Autodesk Inventor part; units mm, degrees
ref_plane "YZ Plane" through (0, 0, 0) normal (1, 0, 0) x (0, 1, 0)
ref_plane "XZ Plane" through (0, 0, 0) normal (0, 1, 0) x (-1, 0, 0)
ref_plane "XY Plane" through (0, 0, 0) normal (0, 0, 1) x (1, 0, 0)
sketch "Sketch23" plane through (0, 0, 0) normal (0, 1, 0) x (-1, 0, 0)
  line L0 (0, -49) -> (0, 49)
  line L1 (49, 0) -> (-49, 0)
  line L2 (35, -35) -> (-35, -35)
  line L3 (-35, -35) -> (-35, 35)
  line L4 (-35, 35) -> (35, 35)
  line L5 (35, 35) -> (35, -35)
  point P0 (0, 0)
  dimension "d310" = 70
  dimension "d311" = 70
extrude "Extrusion14" add sketch "Sketch23" along normal blind 2
sketch "Sketch37" plane through (0, 2, 0) normal (0, 1, 0) x (1, 0, 0)
  line L0 (-35, -35) -> (35, -35)
  line L1 (35, -35) -> (35, 35)
  line L2 (35, 35) -> (-35, 35)
  line L3 (-35, 35) -> (-35, -35)
  line L4 (-49, 0) -> (49, 0)
  line L5 (0, 49) -> (0, -49)
  line L6 (-26.65, 34.3) -> (26.65, 34.3) construction
  line L7 (26.65, 34.3) -> (26.65, -34.3) construction
  line L8 (26.65, -34.3) -> (-26.65, -34.3) construction
  line L9 (-26.65, -34.3) -> (-26.65, 34.3) construction
  point P0 (-24.15, -19)
  point P1 (24.15, -20.3)
  point P2 (19.05, 31.8)
  dimension "d327" = 68.6
  dimension "d328" = 53.3
  dimension "d329" = 15.3
  dimension "d330" = 14
  dimension "d331" = 2.5
  dimension "d332" = 2.5
  dimension "d333" = 2.5
  dimension "d334" = 7.6
hole "Hole18" at (-24.15, 2, 19) at (24.15, 2, 20.3) at (19.05, 2, -31.8) direction (0, -1, 0) diameter 4 end through all
sketch "Sketch40" plane through (0, 2, 0) normal (0, 1, 0) x (1, 0, 0)
  circle A0 centre (19.05, 31.8) radius 2
  circle A1 centre (-24.15, -19) radius 2
  circle A2 centre (24.15, -20.3) radius 2
  line L0 (35, 35) -> (-35, 35)
  line L1 (-35, 35) -> (-35, -35)
  line L2 (-35, -35) -> (35, -35)
  line L3 (35, -35) -> (35, 35)
  line L4 (-49, 0) -> (49, 0)
  line L5 (0, 49) -> (0, -49)
  point P0 (0, 0)
  point P1 (8, 30)
  point P2 (30, 8)
  point P3 (30, -8)
  point P4 (-30, 8)
  point P5 (-30, -8)
  point P6 (-8, -30)
  point P7 (8, -30)
  point P8 (-8, 30)
  dimension "d445" = 8
  dimension "d446" = 5
  dimension "d447" = 8
  dimension "d448" = 5
  dimension "d449" = 8
  dimension "d450" = 5
  dimension "d458" = 8
  dimension "d459" = 8
  dimension "d460" = 5
  dimension "d461" = 5
  dimension "d462" = 5
  dimension "d463" = 8
  dimension "d464" = 8
  dimension "d465" = 5
  dimension "d478" = 8
  dimension "d479" = 5
sketch "Sketch41" plane through (0, 2, 0) normal (0, 1, 0) x (1, 0, 0)
  circle A0 centre (19.05, 31.8) radius 2
  circle A1 centre (-24.15, -19) radius 2
  circle A2 centre (24.15, -20.3) radius 2
  line L0 (35, 35) -> (-35, 35)
  line L1 (-35, 35) -> (-35, -35)
  line L2 (-35, -35) -> (35, -35)
  line L3 (35, -35) -> (35, 35)
  line L4 (-49, 0) -> (49, 0)
  line L5 (0, 49) -> (0, -49)
  line L6 (-20, 20) -> (20, 20)
  line L7 (20, 20) -> (20, 5)
  line L8 (20, 5) -> (-20, 5)
  line L9 (-20, 5) -> (-20, 20)
  line L10 (-20, -5) -> (20, -5)
  line L11 (20, -5) -> (20, -20)
  line L12 (20, -20) -> (-20, -20)
  line L13 (-20, -20) -> (-20, -5)
  dimension "d467" = 10
  dimension "d468" = 40
  dimension "d480" = 15
  dimension "d481" = 15
hole "Hole21" at (8, 2, -30) at (30, 2, -8) at (30, 2, 8) at (-30, 2, -8) at (-30, 2, 8) at (-8, 2, 30) at (8, 2, 30) at (-8, 2, -30) direction (0, -1, 0) diameter 4 end through all
extrude "Extrusion25" cut sketch "Sketch41" against normal up to next contours L6 L7 L8 L5 | L5 L8 L9 L6 | L10 L11 L12 L5 | L5 L12 L13 L10
fillet "Fillet26" radius 6 8 edges at (20, 1, -20) (-20, 1, -20) (-20, 1, -5) (20, 1, -5) (20, 1, 5) (20, 1, 20) (-20, 1, 20) (-20, 1, 5)
chamfer "Chamfer10" distance 12 angle 45 4 edges at (-35, 1, 35) (35, 1, 35) (35, 1, -35) (-35, 1, -35)
fillet "Fillet27" radius 6 8 edges at (-23, 1, 35) (-35, 1, 23) (-35, 1, -23) (-23, 1, -35) (23, 1, -35) (35, 1, -23) (23, 1, 35) (35, 1, 23)
properties part number "body_plate"
The listing builds one solid part. Answer for the finished solid, in the listing's coordinates (mm). A direction names the side the tool comes from. Give positions to 0.01 mm unless a question says otherwise; leave off trailing zeros. Loops run counter-clockwise (first coordinate to the right, second up) from the corner with the lowest first, then second, coordinate; pieces in that order, holes last. Notation, with made-up numbers: (-19, -40) - (-6, -40) arc R3 ccw to (-6, -36) - close; hole circle Ø4 at (-7, -29). An arc over 180 degrees is marked (long way). Return JSON: item names as keys, results as strings. Group by question number.
1. Which of the six approach directions +Z, -Z, +X, -X, +Y, -Y give full straight-line access (tool end or side, diameter ignored) to faces 1 (the cylindrical face through (34.556, 1.014, -22.78)), 2 (the cylindrical face through (18.196, 0.986, -18.289))?
2. Find section B-B (x = 11). Write down the section's boundary in (y, z).
3. Find section A-A (z = 12). Write down the section's boundary in (x, y), then the cut area to 3 significant figures.
4. Find section D-D (x = 19.05). Write down the section's boundary in (y, z).
5. Find section C-C (x = -8). Write down the section's boundary in (y, z), then the cut area to 3 significant figures.
6. Straight lines are drawn through the part: line 1 (Z direction, x = 3, y = 1.3); line 2 (Z direction, x = 30, y = 1.3); line 3 (Z direction, x = 8, y = 0.6). For each, find the intervals that lie inside material, in ascending order. Write a range as [from, to].
7. Given pin 1 Ø1 at (y, z) = (2, -22) entering from -X, flat-ended and moving along its own axis, determine where the tip first touches the part or whether it passes through.
8. Determine the mould class of faces 3 (the cylindrical face through (7.399, 0.986, 31.908)), 4 (the flat face through (0, 0, 0)), 5 (the flat face through (-29, 1, 29)) for opening direction X: pulls with the +X half, pulls with the -X half, needs draft (parallel to the pull), parting line crosses it, or undercut.
Verdict:
{
 "1": {"face 1": "-Z, +X, +Y, -Y", "face 2": "+Y, -Y"},
 "2": {"outline": "(0, -35) - (2, -35) - (2, -20) - (0, -20) - close; (0, -5) - (2, -5) - (2, 5) - (0, 5) - close; (0, 20) - (2, 20) - (2, 35) - (0, 35) - close"},
 "3": {"outline": "(-35, 0) - (-20, 0) - (-20, 2) - (-35, 2) - close; (20, 0) - (35, 0) - (35, 2) - (20, 2) - close", "area": "60.0 mm^2"},
 "4": {"outline": "(0, -35) - (2, -35) - (2, -33.8) - (0, -33.8) - close; (0, -29.8) - (2, -29.8) - (2, -17.24) - (0, -17.24) - close; (0, -7.76) - (2, -7.76) - (2, 7.76) - (0, 7.76) - close; (0, 17.24) - (2, 17.24) - (2, 35) - (0, 35) - close"},
 "5": {"outline": "(0, -35) - (2, -35) - (2, -32) - (0, -32) - close; (0, -28) - (2, -28) - (2, -20) - (0, -20) - close; (0, -5) - (2, -5) - (2, 5) - (0, 5) - close; (0, 20) - (2, 20) - (2, 28) - (0, 28) - close; (0, 32) - (2, 32) - (2, 35) - (0, 35) - close", "area": "64.0 mm^2"},
 "6": {"line 1": "z = [-35, -20], [-5, 5], [20, 35]", "line 2": "z = [-28, -10], [-6, 6], [10, 28]", "line 3": "z = [-35, -32], [-28, -20], [-5, 5], [20, 28], [32, 35]"},
 "7": {"pin 1": "stops at x = -34.92"},
 "8": {"face 3": "undercut", "face 4": "needs draft", "face 5": "pulls with the -X half"}
}
